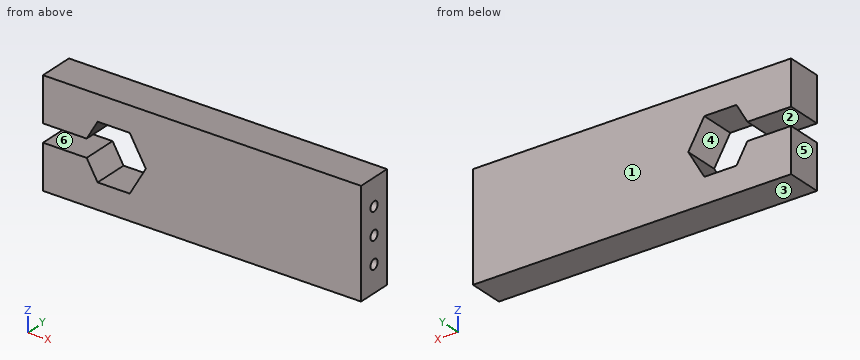
from build123d import *

# Parameters (mm, degrees)
SKETCH1_W                  = 114.3
SKETCH1_H                  = 38.1
BOSS_EXTRUDE1_DEPTH        = 6.35
F_6_32_THREADED_HOLE_D     = 3.5052
F_6_32_THREADED_HOLE_DEPTH = 50.8
F_6_32_THREADED_HOLE_TIP   = 1.053068321
CUT_EXTRUDE1_DEPTH         = 12.7
SKETCH8_W                  = 19.626497308
SKETCH8_H                  = 6.35
CUT_EXTRUDE2_DEPTH         = 117.570504417


with BuildPart() as part:
    # Sketch1 → Boss-Extrude1 (new, symmetric)
    with BuildSketch(Plane(origin=(0, 0, 0), x_dir=(1, 0, 0), z_dir=(0, 1, 0))):
        with Locations((-57.15, 0)):
            Rectangle(SKETCH1_W, SKETCH1_H)
    extrude(amount=BOSS_EXTRUDE1_DEPTH, both=True)

    # #6-32 Threaded Hole
    with Locations(Plane(origin=(0, 0, 0), x_dir=(0, 0, -1), z_dir=(1, 0, 0))):
        with Locations((0, 0), (9.525, 0), (-9.525, 0)):
            Hole(F_6_32_THREADED_HOLE_D / 2, depth=F_6_32_THREADED_HOLE_DEPTH)
            with Locations((0, 0, -(F_6_32_THREADED_HOLE_DEPTH + F_6_32_THREADED_HOLE_TIP / 2))):  # 118° drill point
                Cone(0, F_6_32_THREADED_HOLE_D / 2, F_6_32_THREADED_HOLE_TIP, mode=Mode.SUBTRACT)

    # Sketch5 → Cut-Extrude1 (cut)
    with BuildSketch(Plane(origin=(0, 6.35, 0), x_dir=(1, 0, 0), z_dir=(0, 1, 0))):
        Polygon((-83.126497308, -10), (-77.352994616, 0), (-83.126497308, 10), (-94.673502692, 10), (-100.447005384, 0), (-94.673502692, -10), align=None)
    extrude(amount=-CUT_EXTRUDE1_DEPTH, mode=Mode.SUBTRACT)

    # Sketch8 → Cut-Extrude2 (cut, through all)
    with BuildSketch(Plane(origin=(0, 6.35, 0), x_dir=(1, 0, 0), z_dir=(0, 1, 0))):
        with Locations((-104.486751346, 0)):
            Rectangle(SKETCH8_W, SKETCH8_H)
    extrude(amount=-CUT_EXTRUDE2_DEPTH, mode=Mode.SUBTRACT)


solid = part.part
Work out the finished part from the listing and answer in its coordinate system (mm). Face numbers are marked on the shaded views. A direction names the side the tool comes from. Coordinates: 2 decimals unless noted, no trailing zeros. Write each loop counter-clockwise with the first axis right and the second up, starting at its lowest first coordinate (ties: lowest second). Pieces come first, ordered by that corner, then holes. Notation, with made-up numbers: M -26.5,51.25 L -3.5,51.25 A19 ccw -3.5,75.25 Z; hole C -33.5,25.5 d1. An arc over 180 degrees is marked long. Write item = value, one per line.
1. For the marked faces 4, 5 and 6, determine the directions among +Z, -Z, +X, -X, +Y, -Y from which every point of the face is accessible in a straight line to the end or side of a thin tool.
Solution:
face_4 = +Y, -Y
face_5 = +Z, -Z, -X, +Y, -Y
face_6 = -X, +Y, -Y
2. The part is cut by section A-A (x = -90.5). Determine the outline of the cut face in (y, z).
Solution:
outline = M -6.35,-19.05 L 6.35,-19.05 L 6.35,-10 L -6.35,-10 Z; M -6.35,10 L 6.35,10 L 6.35,19.05 L -6.35,19.05 Z
3. Straight lines are drawn through the part: line 1 (Z direction, x = -28.5, y = 0); line 2 (Z direction, x = -87, y = -1); line 3 (Z direction, x = -41, y = 1.5). For each, find the intervals that lie inside material, in ascending order. Write a range as from..to.
Solution:
line_1 = -19.05..-11.28, -7.77..-1.75, 1.75..7.77, 11.28..19.05
line_2 = -19.05..-10, 10..19.05
line_3 = -19.05..-10.43, -8.62..-0.91, 0.91..8.62, 10.43..19.05
4. The part is cut by section C-C (x = -15). Determine the outline of the cut face in (y, z) (3 decimals), then the cut area to 3 significant figures.
Solution:
outline = M -6.35,-19.05 L 6.35,-19.05 L 6.35,19.05 L -6.35,19.05 Z; hole C 0,-9.525 d3.505; hole C 0,0 d3.505; hole C 0,9.525 d3.505
area = 455 mm2
5. Flat-ended cylindrical pins translate along their axes: pin 1 (3 mm diameter, centred on y = -4.5, z = -8.5, fed in from +X); pin 2 (4 mm diameter, centred on y = 0, z = 0, fed in from -X). Find the tip coordinate at first contact, or state that the pin passes through.
Solution:
pin_1 = 0
pin_2 = -78.51
6. Determine the mould class of the marked faces 1, 2 and 3 for opening direction Z: released by +Z, released by -Z, zero draft, split by the parting line, or undercut.
Solution:
face_1 = zero draft
face_2 = undercut
face_3 = released by -Z
